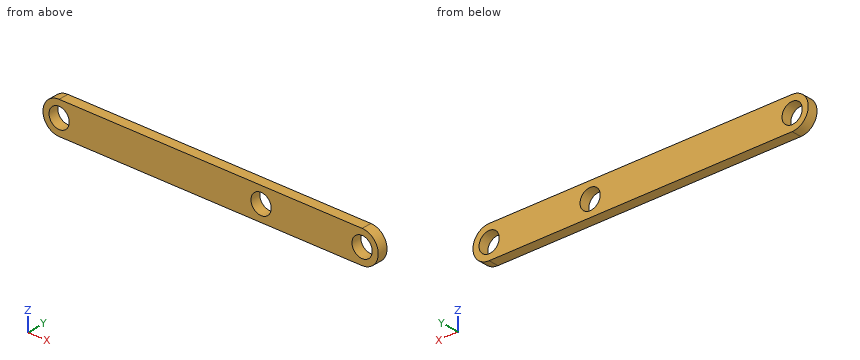
from build123d import *

# Parameters (mm, degrees)
F0_R     = 63.5
F1_DEPTH = 63.5


with BuildPart() as f1:
    # F0 (on Front) → F1 (new body)
    with BuildSketch(Plane.XZ):
        with BuildLine():
            Line((1905, 101.6), (0, 101.6))
            ThreePointArc((0, 101.6), (-101.6, 0), (0, -101.6))
            Line((0, -101.6), (1905, -101.6))
            ThreePointArc((1905, -101.6), (2006.6, 0), (1905, 101.6))
        make_face()
        Circle(F0_R, mode=Mode.SUBTRACT)
        with Locations((1270, 0)):
            Circle(F0_R, mode=Mode.SUBTRACT)
        with Locations((1905, 0)):
            Circle(F0_R, mode=Mode.SUBTRACT)
    extrude(amount=F1_DEPTH)


solid = f1.part
CAD build for the part. Positions are in the model's coordinates, mm. Coordinates: 2 decimals unless noted, no trailing zeros. Write each loop counter-clockwise with the first axis right and the second up, starting at its lowest first coordinate (ties: lowest second). Pieces come first, ordered by that corner, then holes. Notation, with made-up numbers: (74, 39.5) - (93, 39.5) arc R7 cw to (93, 48.5) - close; hole circle Ø3 at (-31.5, 51.5). An arc over 180 degrees is marked (long way). Use a Markdown table: item, result. Add a question column.
Item 1: Drill centre lines: L1, parallel to Z at x = 1905, y = -23; L2, parallel to X at y = -39.5, z = -52.5; L3, parallel to X at y = -31.5, z = 74.5. Where is each one in solid material? Low to high. Write a range as from..to.
Item 2: Flat gauge pins, fed straight in: pin 1 (4 mm diameter, centred on x = 329, z = -79, fed in from +Y); pin 2 (3 mm diameter, centred on y = -33.5, z = -35.5, fed in from +X); pin 3 (1 mm diameter, centred on y = -40.5, z = -6.5, fed in from -X); pin 4 (12 mm diameter, centred on y = -44.5, z = 26, fed in from -X). Where does each tip first touch, or does it go through?
Item 3: Band-saw the part on B-B, the plane x = 1270. Give the cut face in (y, z).
Item 4: Band-saw the part on A-A, the plane z = 0. Give the cut face in (x, y), and give its area (3 significant figures).
Item 5: Band-saw the part on C-C, the plane y = -14. Give the cut face in (x, z).
Numbers:
| question | item | result |
|---|---|---|
| 1 | L1 | -101.6..-63.5, 63.5..101.6 |
| 1 | L2 | -86.98..-35.72, 35.72..1234.28, 1305.72..1869.28, 1940.72..1991.98 |
| 1 | L3 | -69.08..1974.08 |
| 2 | pin 1 | y = 0 |
| 2 | pin 2 | x = 2000.74 |
| 2 | pin 3 | x = -101.42 |
| 2 | pin 4 | x = -99.61 |
| 3 | outline | (-63.5, -101.6) - (0, -101.6) - (0, -63.5) - (-63.5, -63.5) - close; (-63.5, 63.5) - (0, 63.5) - (0, 101.6) - (-63.5, 101.6) - close |
| 4 | outline | (-101.6, -63.5) - (-63.5, -63.5) - (-63.5, 0) - (-101.6, 0) - close; (63.5, -63.5) - (1206.5, -63.5) - (1206.5, 0) - (63.5, 0) - close; (1333.5, -63.5) - (1841.5, -63.5) - (1841.5, 0) - (1333.5, 0) - close; (1968.5, -63.5) - (2006.6, -63.5) - (2006.6, 0) - (1968.5, 0) - close |
| 4 | area | 110,000 mm2 |
| 5 | outline | (0, -101.6) - (1905, -101.6) arc R101.6 ccw to (1905, 101.6) - (0, 101.6) arc R101.6 ccw to start; hole circle Ø127 at (0, 0); hole circle Ø127 at (1270, 0); hole circle Ø127 at (1905, 0) |
